```python
from build123d import *

# Parameters (mm, degrees)
SKETCH1_W                      = 300
SKETCH1_H                      = 300
BOSS_EXTRUDE1_DEPTH            = 20
SKETCH2_W                      = 120
SKETCH2_H                      = 120
CUT_EXTRUDE1_DEPTH             = 214.072757527
CBORE_FOR_M2_SHCS1_D           = 2.4
CBORE_FOR_M2_SHCS1_CBORE_D     = 4.4
CBORE_FOR_M2_SHCS1_CBORE_DEPTH = 2
CBORE_FOR_M2_SHCS2_D           = 2.4
CBORE_FOR_M2_SHCS2_CBORE_D     = 4.4
CBORE_FOR_M2_SHCS2_CBORE_DEPTH = 2
CBORE_FOR_M2_SHCS3_D           = 2.4
CBORE_FOR_M2_SHCS3_CBORE_D     = 4.4
CBORE_FOR_M2_SHCS3_CBORE_DEPTH = 2
SKETCH12_R                     = 20
CUT_EXTRUDE2_DEPTH             = 214.072757527


with BuildPart() as part:
    # Sketch1 → Boss-Extrude1 (new body)
    with BuildSketch(Plane(origin=(0, 0, 0), x_dir=(1, 0, 0), z_dir=(0, 1, 0))):
        Rectangle(SKETCH1_W, SKETCH1_H)
    extrude(amount=BOSS_EXTRUDE1_DEPTH)

    # Sketch2 → Cut-Extrude1 (cut, through all)
    with BuildSketch(Plane(origin=(0, 20, 0), x_dir=(1, 0, 0), z_dir=(0, 1, 0))):
        with Locations((-90, 90)):
            Rectangle(SKETCH2_W, SKETCH2_H)
        with Locations((90, 90)):
            Rectangle(SKETCH2_W, SKETCH2_H)
        with Locations((-90, -90)):
            Rectangle(SKETCH2_W, SKETCH2_H)
        with Locations((90, -90)):
            Rectangle(SKETCH2_W, SKETCH2_H)
    extrude(amount=-CUT_EXTRUDE1_DEPTH, mode=Mode.SUBTRACT)

    # CBORE for M2 SHCS1 (through all)
    with Locations(Plane(origin=(0, 20, 0), x_dir=(1, 0, 0), z_dir=(0, 1, 0))):
        with Locations((-53.93, -22.5), (-107.93, -22.5), (32.88, -12.88), (112.88, -12.88)):
            CounterBoreHole(CBORE_FOR_M2_SHCS1_D / 2, CBORE_FOR_M2_SHCS1_CBORE_D / 2, CBORE_FOR_M2_SHCS1_CBORE_DEPTH)

    # CBORE for M2 SHCS2 (through all)
    with Locations(Plane(origin=(0, 20, 0), x_dir=(1, 0, 0), z_dir=(0, 1, 0))):
        with Locations((22.5, 53.93), (22.5, 107.93), (12.5, -32.88), (12.5, -112.88)):
            CounterBoreHole(CBORE_FOR_M2_SHCS2_D / 2, CBORE_FOR_M2_SHCS2_CBORE_D / 2, CBORE_FOR_M2_SHCS2_CBORE_DEPTH)

    # CBORE for M2 SHCS3 (through all)
    with Locations(Plane(origin=(0, 20, 0), x_dir=(1, 0, 0), z_dir=(0, 1, 0))):
        with Locations((-27.93, 12), (-107.93, 12), (-12, 27.93), (-12, 107.93)):
            CounterBoreHole(CBORE_FOR_M2_SHCS3_D / 2, CBORE_FOR_M2_SHCS3_CBORE_D / 2, CBORE_FOR_M2_SHCS3_CBORE_DEPTH)

    # Sketch12 → Cut-Extrude2 (cut, through all)
    with BuildSketch(Plane(origin=(0, 20, 0), x_dir=(1, 0, 0), z_dir=(0, 1, 0))):
        with Locations(Location((0, 0, 0), (0, 0, 270))):
            Circle(SKETCH12_R)
    extrude(amount=-CUT_EXTRUDE2_DEPTH, mode=Mode.SUBTRACT)


solid = part.part
```
Check sheet for the modelled part. Datum: model origin and axes. Units: mm. A direction names the side the tool comes from. Round coordinates to 2 decimals unless told otherwise and drop trailing zeros. Order: outer loops, then holes, each group sorted by start corner. A loop starts at its lowest first (then second) coordinate and runs counter-clockwise, first axis right, second up. Notation, with made-up numbers: M 38,-22 L 79,-22 A15 cw 79,-6 Z; hole C 20.25,-4.5 d6. An arc over 180 degrees is marked long. Answer in a Markdown table with one row per item.
(1) Material ranges on line 1 along X through (y, z) = (19, 22.5); line 2 along X through (y, z) = (10.75, 22.5); line 3 along X through (y, z) = (14, 113), recorded low to high. Write a range as from..to.
Findings:
| item | result |
|---|---|
| line 1 | x = -150..-110.13, -105.73..-56.13, -51.73..150 |
| line 2 | x = -150..-109.13, -106.73..-55.13, -52.73..150 |
| line 3 | x = -30..11.31, 13.69..30 |
(2) Section check D-D on x = -87. Record the boundary of the cut face in (y, z), plus the area to 3 significant figures.
Findings:
| item | result |
|---|---|
| outline | M 0,-30 L 20,-30 L 20,30 L 0,30 Z |
| area | 1,200 mm^2 |
(3) Gauge pin test, flat ends, axial feed: pin 1 (2.5 mm diameter, centred on x = 22.5, z = -53.93, fed in from -Y); pin 2 (1.3 mm diameter, centred on x = -108.5, z = -11, fed in from +Y); pin 3 (1.5 mm diameter, centred on y = 8.5, z = -97.5, fed in from -X); pin 4 (8 mm diameter, centred on y = 9, z = -42.5, fed in from +X). Record the tip position at first contact, or that the pin passes through.
Findings:
| item | result |
|---|---|
| pin 1 | stops at y = 0 |
| pin 2 | stops at y = 18 |
| pin 3 | stops at x = -30 |
| pin 4 | stops at x = 30 |
(4) Section check A-A on x = 0. Record the boundary of the cut face in (y, z).
Findings:
| item | result |
|---|---|
| outline | M 0,-150 L 20,-150 L 20,-20 L 0,-20 Z; M 0,20 L 20,20 L 20,150 L 0,150 Z |
(5) Section check B-B on y = 5.5. Give the number of separate pieces and of enclosed holes in the cut face, plus the area to 3 significant figures.
Findings:
| item | result |
|---|---|
| separate pieces | 1 |
| enclosed holes | 13 |
| area | 31,100 mm^2 |
(6) Set-up check for faces 1 (the flat face through (89, 10, -30)), 2 (the flat face through (89, 10, 30)), 3 (the flat face through (-1, 0, -23)), 4 (the flat face through (-91, 10, 30)), 5 (the flat face through (-150, 10, 0)): record each of +Z, -Z, +X, -X, +Y, -Y from which the full face is reachable in a straight line by a thin tool's end or side.
Findings:
| item | result |
|---|---|
| face 1 | -Z, +X, +Y, -Y |
| face 2 | +Z, +X, +Y, -Y |
| face 3 | +Z, -Z, +X, -X, -Y |
| face 4 | +Z, -X, +Y, -Y |
| face 5 | +Z, -Z, -X, +Y, -Y |
(7) Section check C-C on z = 78.5. Record the boundary of the cut face in (x, y).
Findings:
| item | result |
|---|---|
| outline | M -30,0 L 30,0 L 30,20 L -30,20 Z |
(8) Draft check along Z on faces 6 (the flat face through (0, 10, 150)), 7 (the cylindrical face through (-19.524, 10.14, -4.336)), 8 (the flat face through (-30, 10, -89)), 9 (the flat face through (-91, 10, -30)). Enter one of: +Z half, -Z half, draft (parallel to the pull), parting line (faces both ways), or undercut.
Findings:
| item | result |
|---|---|
| face 6 | +Z half |
| face 7 | undercut |
| face 8 | draft |
| face 9 | -Z half |
